Design review of the part built by this model. Coordinates are the model's own, in mm. Round coordinates to 2 decimals unless told otherwise and drop trailing zeros. Write each loop counter-clockwise with the first axis right and the second up, starting at its lowest first coordinate (ties: lowest second). Pieces come first, ordered by that corner, then holes. Notation, with made-up numbers: (-13.5, 47.5) -> (-0.5, 47.5) arc R26 ccw to (-0.5, 79.5) -> close; hole circle Ø8 at (6, 52.25). An arc over 180 degrees is marked (long way). Write item = value, one per line. Start each with the question number.
Item 1: Add section C-C, the plane x = 24. State the section outline as (y, z) points (3 decimals).
Item 2: Add section B-B, the plane z = 1.2. State how many separate pieces and enclosed holes the cut face has, then the cut area to 3 significant figures.
Item 3: To check wall thickness, follow L1, parallel to X at y = 6.5, z = 2.65; L2, parallel to Y at x = 44.45, z = 0.8; L3, parallel to Y at x = 24.5, z = 1.85. State the ranges of each line that lie inside material, in increasing order.
Item 4: For pin 1 Ø1 at (x, z) = (34.5, 2.5) entering from +Y; pin 2 Ø1.5 at (y, z) = (27, 1) entering from -X; pin 3 Ø3 at (x, y) = (8.33, 6.35) entering from -Z, all flat-tipped, find the tip position at first contact; note any pin that passes through.
Item 5: Add section A-A, the plane x = 43.5. State the section outline as (y, z) points (3 decimals).
Item 6: Add section D-D, the plane x = 9. State the section outline as (y, z) points (3 decimals).
from build123d import *

# Parameters (mm, degrees)
F0_R     = 2.38125
F1_DEPTH = 3.175
F2_R     = 6.34999


# Not quite as in the source:
# - a fillet or chamfer is up to 0.001 mm smaller than in the source, because OpenCascade refuses the exact size


with BuildPart() as f1:
    # F0 (on Top) → F1 (new body)
    with BuildSketch(Plane.XY):
        Polygon((0, 12.7), (0, 0), (50.8, 0), (50.8, 50.8), (38.1, 50.8), (38.1, 12.7), align=None)
        with Locations((8.3286329803, 6.35)):
            Circle(F0_R, mode=Mode.SUBTRACT)
        with Locations((44.45, 42.4713670197)):
            Circle(F0_R, mode=Mode.SUBTRACT)
    extrude(amount=F1_DEPTH)

    # F2 (radius 6.35 in the source; OpenCascade refuses exactly that, so slightly less here)
    f2_edges = [f1.edges().sort_by_distance(p)[0] for p in [
        (0, 0, 1.5875),
        (0, 12.7, 1.5875),
        (38.1, 50.8, 1.5875),
        (38.1, 12.7, 1.5875),
        (50.8, 0, 1.5875),
        (50.8, 50.8, 1.5875),
    ]]
    fillet(f2_edges, radius=F2_R)


solid = f1.part
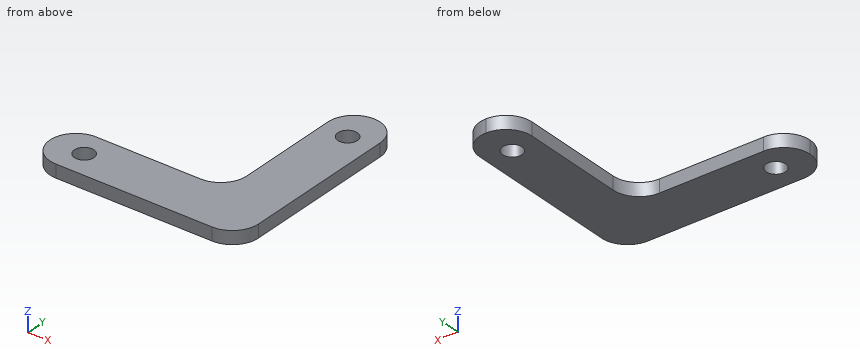
Result set:
q1.outline = (0, 0) -> (12.7, 0) -> (12.7, 3.175) -> (0, 3.175) -> close
q2.separate_pieces = 1
q2.enclosed_holes = 2
q2.area = 1,060 mm²
q3.L1 = 0 to 5.95, 10.71 to 50.8
q3.L2 = 0 to 40.09, 44.85 to 50.8
q3.L3 = 0 to 12.7
q4.pin_1 = 13.59
q4.pin_2 = 38.1
q4.pin_3 = through
q5.outline = (0, 0) -> (40.288, 0) -> (40.288, 3.175) -> (0, 3.175) -> close; (44.655, 0) -> (50.729, 0) -> (50.729, 3.175) -> (44.655, 3.175) -> close
q6.outline = (0, 0) -> (4.065, 0) -> (4.065, 3.175) -> (0, 3.175) -> close; (8.635, 0) -> (12.7, 0) -> (12.7, 3.175) -> (8.635, 3.175) -> close
